```python
from build123d import *

# Parameters (mm, degrees)
F0_R     = 2
F0_W     = 40
F0_H     = 25
F1_DEPTH = 2
F3_START = -10
F3_DEPTH = 43
F4_R     = 1
F5_R     = 7.5
F5_R_2   = 2
F6_DEPTH = 2
F7_SIZE  = 2


with BuildPart() as f1:
    # F0 (on Front) → F1 (new body)
    with BuildSketch(Plane.XZ):
        Polygon((62.25, 29.75), (-62.25, 29.75), (-62.25, -29.75), (-13.75, -29.75), (-13.75, -31.25), (5.75, -31.25), (5.75, -29.75), (62.25, -29.75), align=None)
        with Locations((-42.25, 0)):
            Circle(F0_R, mode=Mode.SUBTRACT)
        Rectangle(F0_W, F0_H, mode=Mode.SUBTRACT)
        with Locations((42.25, 0)):
            Circle(F0_R, mode=Mode.SUBTRACT)
    extrude(amount=F1_DEPTH)

    # F2 (on face) → F3 (join)
    with BuildSketch(Plane(origin=(0, 0, -29.75), x_dir=(1, 0, 0), z_dir=(0, 0, -1)).offset(F3_START)):
        Polygon((-61.25, 12), (-61.25, 2), (-60.25, 2), (-60.25, 18.1445069205), (-62.25, 16.1445069205), (-62.25, 14.1445069205), align=None)
        Polygon((61.25, 2), (61.25, 12), (62.25, 14.1445069205), (62.25, 16.1445069205), (60.25, 18.1445069205), (60.25, 2), align=None)
    extrude(amount=-F3_DEPTH)

    # F4
    f4_edges = [f1.edges().sort_by_distance(p)[0] for p in [
        (-62.25, -1, -29.75),
        (62.25, -1, -29.75),
        (62.25, -1, 29.75),
        (-62.25, -1, 29.75),
    ]]
    fillet(f4_edges, radius=F4_R)

    # F5 (on face) → F6 (join)
    with BuildSketch(Plane.XZ.offset(2)):
        with Locations((-42.25, 0)):
            Circle(F5_R)
        with Locations((-42.25, 0)):
            Circle(F5_R_2, mode=Mode.SUBTRACT)
        with Locations((42.25, 0)):
            Circle(F5_R)
        with Locations((42.25, 0)):
            Circle(F5_R_2, mode=Mode.SUBTRACT)
    extrude(amount=F6_DEPTH)

    # F7
    f7_edges = [f1.edges().sort_by_distance(p)[0] for p in [
        (-44.25, -4, 0),
        (40.25, -4, 0),
    ]]
    chamfer(f7_edges, length=F7_SIZE)


solid = f1.part
```
Can you work these out from the model? Positions are in its coordinate system, mm. A direction names the side the tool comes from. Round coordinates to 2 decimals unless told otherwise and drop trailing zeros. Loops run counter-clockwise (first coordinate to the right, second up) from the corner with the lowest first, then second, coordinate; pieces in that order, holes last. Notation, with made-up numbers: (72, 36) -> (104, 36) arc R23 ccw to (104, 55) -> close; hole circle Ø11 at (78, 16.25). An arc over 180 degrees is marked (long way). One line per item, written item: value. Start each with the question number.
1. If I drill on probe 1 along Z at (x, y) = (-42.25, -0.7); probe 2 along X at (y, z) = (-14.75, -1); probe 3 along X at (y, z) = (-11.25, 6), over which ranges is the centre line in solid material (lowest first)?
2. If we mould it in two halves opening along Y, with no side actions, what happens to faces 6 (the flat face through (60.25, -10, 1)), 7 (the flat face through (61.25, -7, 1)), 8 (the flat face through (45.5, -4, -3.2))? For each: pulls with the +Y half, pulls with the -Y half, needs draft (parallel to the pull), parting line crosses it, or undercut.
3. If we section it at D-D, the plane z = 21: Write out the boundary of the cut face in (x, y).
4. For faces 1 (the flat face through (-61.25, -7, 1)), 2 (the cylindrical face through (-35.096, -2.986, 2.253)), 3 (the flat face through (61.743, -13.057, 1.449)), 4 (the flat face through (-39, -4, -3)), 5 (the flat face through (-1, 0, -14)), which set-ups out of +Z, -Z, +X, -X, +Y, -Y let a thin tool reach every point of the face, with its end or its side?
5. If we section it at C-C, the plane x = 42.25: Write out the boundary of the cut face in (y, z).
6. If we section it at B-B, the plane y = -10.25: Write out the boundary of the cut face in (x, z), then the cut area to 3 significant figures.
7. For pin 1 (5 mm diameter, centred on y = -8.5, z = 0, fed in from -X); pin 2 (4.5 mm diameter, centred on x = -42.25, z = 0, fed in from -Y); pin 3 (1 mm diameter, centred on x = -61, y = -7.5, fed in from -Z), each with a flat end and sliding along its axis, tell me the tip position at first contact or that it passes through.
8. If we section it at A-A, the plane z = 6: Write out the boundary of the cut face in (x, y), then the cut area to 3 significant figures.
Calculated:
1. probe 1: z = -29.75 to -2, 2 to 29.75
1. probe 2: x = -62.25 to -60.25, 60.25 to 62.25
1. probe 3: x = -61.25 to -60.25, 60.25 to 61.25
2. face 6: needs draft
2. face 7: undercut
2. face 8: pulls with the -Y half
3. outline: (-62.25, -16.14) -> (-60.25, -18.14) -> (-60.25, -2) -> (60.25, -2) -> (60.25, -18.14) -> (62.25, -16.14) -> (62.25, -14.14) -> (61.25, -12) -> (61.25, -2) -> (62.25, -2) -> (62.25, 0) -> (-62.25, 0) -> (-62.25, -2) -> (-61.25, -2) -> (-61.25, -12) -> (-62.25, -14.14) -> close
4. face 1: +Z, -Z, -X
4. face 2: -Y
4. face 3: +Z, -Z, +X
4. face 4: +Z, -Z, -Y
4. face 5: +Z, -Z, +X, -X, +Y
5. outline: (-4, -7.5) -> (-2, -7.5) -> (-2, -29.75) -> (0, -29.75) -> (0, -2) -> (-2, -2) -> (-4, -4) -> close; (-4, 4) -> (-2, 2) -> (0, 2) -> (0, 29.75) -> (-2, 29.75) -> (-2, 7.5) -> (-4, 7.5) -> close
6. outline: (-61.25, -19.75) -> (-60.25, -19.75) -> (-60.25, 23.25) -> (-61.25, 23.25) -> close; (60.25, -19.75) -> (61.25, -19.75) -> (61.25, 23.25) -> (60.25, 23.25) -> close
6. area: 86.0 mm²
7. pin 1: stops at x = -61.25
7. pin 2: stops at y = -2.25
7. pin 3: stops at z = -19.75
8. outline: (-62.25, -16.14) -> (-60.25, -18.14) -> (-60.25, -2) -> (-46.75, -2) -> (-46.75, -4) -> (-37.75, -4) -> (-37.75, -2) -> (-20, -2) -> (-20, 0) -> (-62.25, 0) -> (-62.25, -2) -> (-61.25, -2) -> (-61.25, -12) -> (-62.25, -14.14) -> close; (20, -2) -> (37.75, -2) -> (37.75, -4) -> (46.75, -4) -> (46.75, -2) -> (60.25, -2) -> (60.25, -18.14) -> (62.25, -16.14) -> (62.25, -14.14) -> (61.25, -12) -> (61.25, -2) -> (62.25, -2) -> (62.25, 0) -> (20, 0) -> close
8. area: 243 mm²
